from build123d import *

# Parameters (mm, degrees)
SKETCH_R        = 25.999973
PAD_DEPTH       = 2
SKETCH001_R     = 1.5
POCKET_DEPTH    = 2.001
SKETCH002_W     = 21
SKETCH002_H     = 13.007144
POCKET001_DEPTH = 5
FILLET_R        = 2


with BuildPart() as part:
    # Sketch → Pad (new body)
    with BuildSketch(Plane.XY):
        Circle(SKETCH_R)
    extrude(amount=PAD_DEPTH)

    # Sketch001 (on Face3 of Pad) → Pocket (cut, through all)
    with BuildSketch(Plane.XY.offset(2)):
        with Locations((-15, 15)):
            Circle(SKETCH001_R)
        with Locations((15, 15)):
            Circle(SKETCH001_R)
        with Locations((15, -15)):
            Circle(SKETCH001_R)
        with Locations((-15, -15)):
            Circle(SKETCH001_R)
    extrude(amount=-POCKET_DEPTH, mode=Mode.SUBTRACT)

    # Sketch002 (on Face3 of Pocket) → Pocket001 (cut)
    with BuildSketch(Plane.XY.offset(2)):
        with Locations((15.5, -0.003572)):
            Rectangle(SKETCH002_W, SKETCH002_H)
    extrude(amount=-POCKET001_DEPTH, mode=Mode.SUBTRACT)

    # Fillet
    fillet_edges = [part.edges().sort_by_distance(p)[0] for p in [
        (5, 6.5, 1),
        (5, -6.507144, 1),
        (25.172518, -6.507144, 1),
        (25.174364, 6.5, 1),
    ]]
    fillet(fillet_edges, radius=FILLET_R)


solid = part.part
Here's how the part is built. I have some questions about the finished solid (model axes, mm). A direction names the side the tool comes from. Give positions to 0.01 mm unless a question says otherwise; leave off trailing zeros. Order: outer loops, then holes, each group sorted by start corner. A loop starts at its lowest first (then second) coordinate and runs counter-clockwise, first axis right, second up. Notation, with made-up numbers: (70, -4) -> (94, -4) arc R25 ccw to (94, 26) -> close; hole circle Ø9 at (-5.5, -30). An arc over 180 degrees is marked (long way). Use a Markdown table: item, result. Add a question column.
Item 1: Will these pins go through, and if not, where does the flat tip stop? pin 1 (0.6 mm diameter, centred on x = 13, z = 1, fed in from -Y); pin 2 (12 mm diameter, centred on x = 14.5, y = -9, fed in from -Z).
Item 2: I need wall thicknesses on line 1 (Y direction, x = -15, z = 1.55); line 2 (Y direction, x = 15, z = 1.4); line 3 (X direction, y = 15.5, z = 1.6). Which ranges of each line are inside material? Lowest first, please.
Item 3: Imagine slicing it at B-B on z = 0.75. Please give me the cut outline in (x, y), plus the area to 3 significant figures.
Item 4: For faces 1 (the face through (-25.98, 1.02, 0.99)), 2 (the face through (15, 6.5, 1)), which set-ups out of +Z, -Z, +X, -X, +Y, -Y let a thin tool reach every point of the face, with its end or its side?
Item 5: If we mould it in two halves opening along X, with no side actions, what happens to faces 3 (the face through (13.5, -14.93, 1.01)), 4 (the face through (-1, 0, 2)), 5 (the face through (-16.5, -14.93, 1.01)), 6 (the face through (5.601, -5.937, 0.986))? For each: pulls with the +X half, pulls with the -X half, needs draft (parallel to the pull), parting line crosses it, or undercut.
Item 6: Imagine slicing it at A-A on x = -15. Please give me the cut outline in (y, z).
Item 7: Imagine slicing it at C-C on x = 15. Please give me the cut outline in (y, z), plus the area to 3 significant figures.
Data:
| question | item | result |
|---|---|---|
| 1 | pin 1 | stops at y = -22.69 |
| 1 | pin 2 | stops at z = 0 |
| 2 | line 1 | y = -21.24 to -16.5, -13.5 to 13.5, 16.5 to 21.24 |
| 2 | line 2 | y = -21.24 to -16.5, -13.5 to -6.51, 6.5 to 13.5, 16.5 to 21.24 |
| 2 | line 3 | x = -20.87 to -16.41, -13.59 to 13.59, 16.41 to 20.87 |
| 3 | outline | (5, -4.51) -> (5, 4.5) arc R2 cw to (7, 6.5) -> (22.44, 6.5) arc R2 ccw to (24.31, 9.21) arc R26 ccw (long way) to (24.31, -9.22) arc R2 ccw to (22.44, -6.51) -> (7, -6.51) arc R2 cw to start; hole circle Ø3 at (-15, -15); hole circle Ø3 at (-15, 15); hole circle Ø3 at (15, -15); hole circle Ø3 at (15, 15) |
| 3 | area | 1,820 mm² |
| 4 | face 1 | +Z, -Z |
| 4 | face 2 | +Z, -Z, +X |
| 5 | face 3 | undercut |
| 5 | face 4 | needs draft |
| 5 | face 5 | undercut |
| 5 | face 6 | pulls with the +X half |
| 6 | outline | (-21.24, 0) -> (-16.5, 0) -> (-16.5, 2) -> (-21.24, 2) -> close; (-13.5, 0) -> (13.5, 0) -> (13.5, 2) -> (-13.5, 2) -> close; (16.5, 0) -> (21.24, 0) -> (21.24, 2) -> (16.5, 2) -> close |
| 7 | outline | (-21.24, 0) -> (-16.5, 0) -> (-16.5, 2) -> (-21.24, 2) -> close; (-13.5, 0) -> (-6.51, 0) -> (-6.51, 2) -> (-13.5, 2) -> close; (6.5, 0) -> (13.5, 0) -> (13.5, 2) -> (6.5, 2) -> close; (16.5, 0) -> (21.24, 0) -> (21.24, 2) -> (16.5, 2) -> close |
| 7 | area | 46.9 mm² |
